```python
from build123d import *

# Parameters (mm, degrees)
BOSS_EXTRUDE1_DEPTH     = 110
CUT_EXTRUDE1_DEPTH      = 1
CUT_EXTRUDE1_DEPTH_BACK = 111
SKETCH4_R               = 3
CUT_EXTRUDE2_DEPTH      = 1
CUT_EXTRUDE2_DEPTH_BACK = 43.893018073
BOSS_EXTRUDE2_DEPTH     = 30
SKETCH6_W               = 26.1276751
SKETCH6_H               = 29.954556473
CUT_EXTRUDE3_DEPTH      = 19.975306871
CUT_EXTRUDE3_DEPTH_BACK = 30.07458706


with BuildPart() as part:
    # Sketch1 → Boss-Extrude1 (new body)
    with BuildSketch(Plane.XY):
        Polygon((0, 0), (-142.475314215, -32.893018073), (-143.119166497, -30.104187448), (-118.522600871, -18.772135805), align=None)
    extrude(amount=BOSS_EXTRUDE1_DEPTH)

    # Sketch2 → Cut-Extrude1 (cut, two sides)
    with BuildSketch(Plane.XY.offset(110)) as cut_extrude1_sk:
        Polygon((-21.820404963, -3.456012628), (-21.820404963, -5.037637423), (0, 0), align=None)
    extrude(amount=CUT_EXTRUDE1_DEPTH, mode=Mode.SUBTRACT)
    extrude(cut_extrude1_sk.sketch, amount=-CUT_EXTRUDE1_DEPTH_BACK, mode=Mode.SUBTRACT)

    # Sketch4 → Cut-Extrude2 (cut, two sides)
    with BuildSketch(Plane(origin=(0, 10, 0), x_dir=(1, 0, 0), z_dir=(0, 1, 0))) as cut_extrude2_sk:
        with Locations((-130.995623221, -101)):
            Circle(SKETCH4_R)
        with Locations((-131.538244407, -9)):
            Circle(SKETCH4_R)
        with Locations((-130.995623221, -55)):
            Circle(SKETCH4_R)
        with BuildLine():
            Line((-29.820404963, -105), (-109.820404963, -105))
            ThreePointArc((-109.820404963, -105), (-113.820404963, -101), (-109.820404963, -97))
            Line((-109.820404963, -97), (-29.820404963, -97))
            ThreePointArc((-29.820404963, -97), (-25.820404963, -101), (-29.820404963, -105))
        make_face()
        with BuildLine():
            Line((-29.820404963, -5), (-109.820404963, -5))
            ThreePointArc((-109.820404963, -5), (-113.820404963, -9), (-109.820404963, -13))
            Line((-109.820404963, -13), (-29.820404963, -13))
            ThreePointArc((-29.820404963, -13), (-25.820404963, -9), (-29.820404963, -5))
        make_face()
    extrude(amount=CUT_EXTRUDE2_DEPTH, mode=Mode.SUBTRACT)
    extrude(cut_extrude2_sk.sketch, amount=-CUT_EXTRUDE2_DEPTH_BACK, mode=Mode.SUBTRACT)

    # Sketch5 → Boss-Extrude2 (add)
    with BuildSketch(Plane.XY.offset(110)):
        Polygon((-142.475314215, -32.893018073), (-21.820404963, -5.037637423), (-21.820404963, -3.456012628), (-118.522600871, -18.772135805), (-143.119166497, -30.104187448), align=None)
    extrude(amount=BOSS_EXTRUDE2_DEPTH)

    # Sketch6 → Cut-Extrude3 (cut, two sides)
    with BuildSketch(Plane(origin=(0, 0, 0), x_dir=(0.987688341, 0.156434465, 0), z_dir=(-0.156434465, 0.987688341, 0))) as cut_extrude3_sk:
        with BuildLine():
            Line((-30.192120061, -134.324079108), (-111.189330125, -134.324079108))
            ThreePointArc((-111.189330125, -134.324079108), (-115.189330125, -130.324079108), (-111.189330125, -126.324079108))
            Line((-111.189330125, -126.324079108), (-30.192120061, -126.324079108))
            ThreePointArc((-30.192120061, -126.324079108), (-26.192120061, -130.324079108), (-30.192120061, -134.324079108))
        make_face()
        with Locations((-133.06383755, -125.022721764)):
            Rectangle(SKETCH6_W, SKETCH6_H)
    extrude(amount=CUT_EXTRUDE3_DEPTH, mode=Mode.SUBTRACT)
    extrude(cut_extrude3_sk.sketch, amount=-CUT_EXTRUDE3_DEPTH_BACK, mode=Mode.SUBTRACT)


solid = part.part
```
The model under review builds one solid part; all positions refer to its coordinate system, in mm. A direction names the side the tool comes from. Give positions to 0.01 mm unless a question says otherwise; leave off trailing zeros. Loops run counter-clockwise (first coordinate to the right, second up) from the corner with the lowest first, then second, coordinate; pieces in that order, holes last. Notation, with made-up numbers: (76, 87.5) - (126, 87.5) arc R23 ccw to (126, 103.5) - close; hole circle Ø5 at (42, -33.5). An arc over 180 degrees is marked (long way). Answer as a JSON object with one key per item and string values.
Q1. Add section B-B on z = 55. State the section outline as (x, y) points, plus the area to 3 significant figures.
Worked out:
{"outline": "(-143.12, -30.1) - (-142.48, -32.89) - (-134, -30.94) - (-134, -25.9) - close; (-128, -29.55) - (-21.82, -5.04) - (-21.82, -3.46) - (-118.52, -18.77) - (-128, -23.14) - close", "area": "598 mm^2"}
Q2. Insertion check: pin 1 (15.5 mm diameter, centred on x = -133.5, y = -22.5, fed in from +Z); pin 2 (5 mm diameter, centred on x = -35.5, z = 51.5, fed in from -Y); pin 3 (2 mm diameter, centred on x = -130.5, z = 32.5, fed in from -Y); pin 4 (5.5 mm diameter, centred on x = -131.54, z = 9, fed in from +Y). Each pin has a flat end and moves straight along its axis. Give the tip position at first contact, or say it passes through.
Worked out:
{"pin 1": "stops at z = 110.05", "pin 2": "stops at y = -8.77", "pin 3": "stops at y = -30.36", "pin 4": "passes through"}
Q3. For faces 1 (the cylindrical face through (-113.145, -21.969, 130.412)), 2 (the flat face through (-117.875, -22.858, 125.232)), list the 3-axis set-ups (+Z, -Z, +X, -X, +Y, -Y) from which the entire face can be reached by the end or side of a thin tool; tool diameter is ignored.
Worked out:
{"face 1": "+X, +Y", "face 2": "+Z, -X, -Y"}
Q4. To check wall thickness, follow line 1 along Z through (x, y) = (-100, -21.5); line 2 along Z through (x, y) = (-135.5, -27.5); line 3 along X through (y, z) = (-26, 9). State the ranges of each line that lie inside material, in increasing order.
Worked out:
{"line 1": "z = 0 to 5, 13 to 97, 105 to 126.32, 134.32 to 140", "line 2": "z = 0 to 110.05", "line 3": "x = -128.54 to -113.82"}
Q5. Add section D-D on z = 9. State the section outline as (x, y) points, plus the area to 3 significant figures.
Worked out:
{"outline": "(-143.12, -30.1) - (-142.48, -32.89) - (-134.54, -31.06) - (-134.54, -26.15) - close; (-128.54, -29.68) - (-113.82, -26.28) - (-113.82, -18.03) - (-118.52, -18.77) - (-128.54, -23.39) - close; (-25.82, -5.96) - (-21.82, -5.04) - (-21.82, -3.46) - (-25.82, -4.09) - close", "area": "154 mm^2"}
Q6. Add section A-A on x = -70.5. State the section outline as (y, z) points.
Worked out:
{"outline": "(-16.28, 0) - (-11.17, 0) - (-11.17, 5) - (-16.28, 5) - close; (-16.28, 13) - (-11.17, 13) - (-11.17, 97) - (-16.28, 97) - close; (-16.28, 105) - (-11.17, 105) - (-11.17, 126.32) - (-16.28, 126.32) - close; (-16.28, 134.32) - (-11.17, 134.32) - (-11.17, 140) - (-16.28, 140) - close"}
Q7. Mouldability with a two-part tool opening along Z and no side actions: class faces 3 (the flat face through (-81, -16, 140)), 4 (the flat face through (-91, -18, 0)), 5 (the cylindrical face through (-128.677, -27.202, 8.099)) as +Z half, -Z half, draft (parallel to the pull), parting line (faces both ways), or undercut.
Worked out:
{"face 3": "+Z half", "face 4": "-Z half", "face 5": "undercut"}
Q8. Add section C-C on y = -10.25. State the section outline as (x, z) points.
Worked out:
{"outline": "(-64.72, 0) - (-44.4, 0) - (-44.4, 5) - (-64.72, 5) - close; (-64.72, 13) - (-44.4, 13) - (-44.4, 97) - (-64.72, 97) - close; (-64.72, 105) - (-44.4, 105) - (-44.4, 126.32) - (-64.72, 126.32) - close; (-64.72, 134.32) - (-44.4, 134.32) - (-44.4, 140) - (-64.72, 140) - close"}
